For this review, use the dimensioned drawing (mm, ordinates from the lowest corner) and the shaded views. A direction names the side the tool comes from. Give positions to 0.01 mm unless a question says otherwise; leave off trailing zeros. Order: outer loops, then holes, each group sorted by start corner. A loop starts at its lowest first (then second) coordinate and runs counter-clockwise, first axis right, second up.
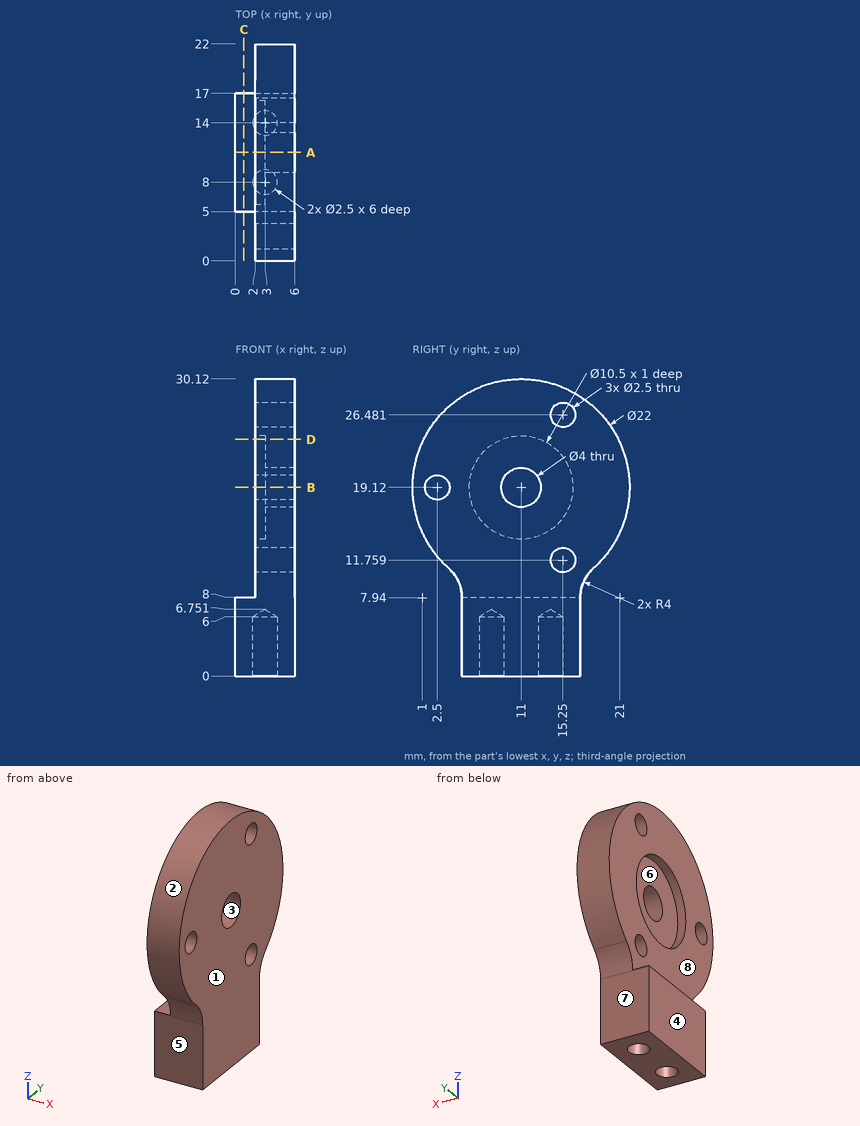
1. Take a section at D-D (z = 24). Write out the cut boundary in (x, y), and give its area (3 significant figures).
2. For the marked faces 4, 5, 6, 7 and 8, list the 3-axis set-ups (+Z, -Z, +X, -X, +Y, -Y) from which the entire face can be reached by the end or side of a thin tool; tool diameter is ignored.
3. Take a section at B-B (z = 19.12). Write out the cut boundary in (x, y).
4. To check wall thickness, follow line 1 (Z direction, x = 4.25, y = 15.25) (1 decimal); line 2 (Z direction, x = 5.1, y = 11); line 3 (Y direction, x = 2.2, z = 4.5). State the ranges of each line that lie inside material, in increasing order.
5. Insertion check: pin 1 (1 mm diameter, centred on y = 6, z = 17.5, fed in from -X); pin 2 (2 mm diameter, centred on x = 3, y = 14, fed in from -Z); pin 3 (1 mm diameter, centred on x = 2.5, y = 14, fed in from +Z); pin 4 (3 mm diameter, centred on x = 3, y = 8, fed in from -Z). Each pin has a flat end and moves straight along its axis. Give the tip position at first contact, or say it passes through.
6. Draft analysis for pull direction Z (two halves, no side actions). For the marked faces 1, 2 and 3, state which applies: pulls with the +Z half, pulls with the -Z half, needs draft (parallel to the pull), parting line crosses it, or undercut.
7. Take a section at C-C (x = 0.85). Write out the cut boundary in (y, z), and give its area (3 significant figures).
8. Take a section at A-A (y = 11). Write out the cut boundary in (x, z).
Answer:
1. outline: (2, 1.14) - (6, 1.14) - (6, 20.86) - (2, 20.86) - (2, 12.94) - (3, 12.94) - (3, 9.06) - (2, 9.06) - close
1. area: 75.0 mm2
2. face 4: +Z, -Z, -X, +Y, -Y
2. face 5: -Z, +X, -X, -Y
2. face 6: -X
2. face 7: -Z, +X, -X, +Y
2. face 8: +Z, -X, +Y, -Y
3. outline: (2, 0) - (6, 0) - (6, 1.25) - (2, 1.25) - close; (2, 3.75) - (6, 3.75) - (6, 9) - (3, 9) - (3, 5.75) - (2, 5.75) - close; (2, 16.25) - (3, 16.25) - (3, 13) - (6, 13) - (6, 22) - (2, 22) - close
4. line 1: z = 0 to 10.5, 13 to 25.2, 27.7 to 29.3
4. line 2: z = 0 to 17.12, 21.12 to 30.12
4. line 3: y = 5 to 7.04, 8.96 to 13.04, 14.96 to 17
5. pin 1: stops at x = 2
5. pin 2: stops at z = 6.15
5. pin 3: stops at z = 29.83
5. pin 4: stops at z = 0
6. face 1: needs draft
6. face 2: parting line crosses it
6. face 3: undercut
7. outline: (5, 0) - (17, 0) - (17, 7.94) arc R4 cw to (17, 8) - (5, 8) arc R4 cw to (5, 7.94) - close
7. area: 96.0 mm2
8. outline: (0, 0) - (6, 0) - (6, 17.12) - (3, 17.12) - (3, 13.87) - (2, 13.87) - (2, 8) - (0, 8) - close; (2, 24.37) - (3, 24.37) - (3, 21.12) - (6, 21.12) - (6, 30.12) - (2, 30.12) - close
